```python
from build123d import *

# Parameters (mm, degrees)
SKETCH1_W           = 203.2
SKETCH1_H           = 152.4
BOSS_EXTRUDE1_DEPTH = 3.175


with BuildPart() as part:
    # Sketch1 → Boss-Extrude1 (new body)
    with BuildSketch(Plane(origin=(0, 0, 0), x_dir=(1, 0, 0), z_dir=(0, 1, 0))):
        with Locations((12.7, 0)):
            Rectangle(SKETCH1_W, SKETCH1_H)
        with BuildLine():
            Line((-48.396184338, 37.144491245), (-40.325508755, 43.316184338))
            ThreePointArc((-40.325508755, 43.316184338), (-33.204324417, 42.366693093), (-34.153815662, 35.245508755))
            Line((-34.153815662, 35.245508755), (-42.224491245, 29.073815662))
            ThreePointArc((-42.224491245, 29.073815662), (-49.345675583, 30.023306907), (-48.396184338, 37.144491245))
        make_face(mode=Mode.SUBTRACT)
        with BuildLine():
            Line((34.153815662, 35.245508755), (42.224491245, 29.073815662))
            ThreePointArc((42.224491245, 29.073815662), (49.345675583, 30.023306907), (48.396184338, 37.144491245))
            Line((48.396184338, 37.144491245), (40.325508755, 43.316184338))
            ThreePointArc((40.325508755, 43.316184338), (33.204324417, 42.366693093), (34.153815662, 35.245508755))
        make_face(mode=Mode.SUBTRACT)
        with BuildLine():
            Line((34.153815662, -35.245508755), (42.224491245, -29.073815662))
            ThreePointArc((42.224491245, -29.073815662), (49.345675583, -30.023306907), (48.396184338, -37.144491245))
            Line((48.396184338, -37.144491245), (40.325508755, -43.316184338))
            ThreePointArc((40.325508755, -43.316184338), (33.204324417, -42.366693093), (34.153815662, -35.245508755))
        make_face(mode=Mode.SUBTRACT)
        with BuildLine():
            Line((-48.396184338, -37.144491245), (-40.325508755, -43.316184338))
            ThreePointArc((-40.325508755, -43.316184338), (-33.204324417, -42.366693093), (-34.153815662, -35.245508755))
            Line((-34.153815662, -35.245508755), (-42.224491245, -29.073815662))
            ThreePointArc((-42.224491245, -29.073815662), (-49.345675583, -30.023306907), (-48.396184338, -37.144491245))
        make_face(mode=Mode.SUBTRACT)
    extrude(amount=BOSS_EXTRUDE1_DEPTH)


solid = part.part
```
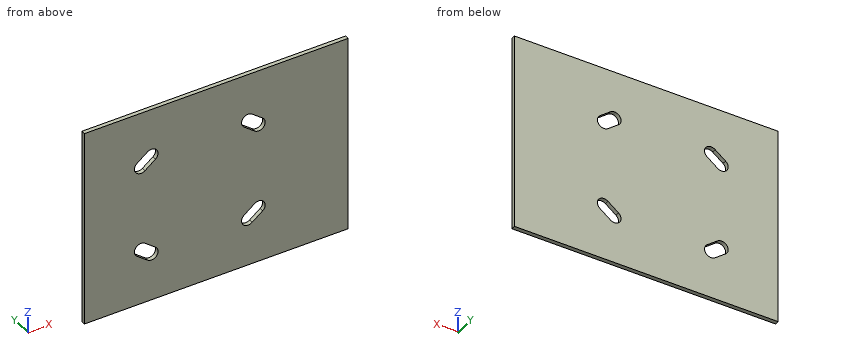
The listing builds one solid part. Answer for the finished solid, in the listing's coordinates (mm). Coordinates: 2 decimals unless noted, no trailing zeros. Write each loop counter-clockwise with the first axis right and the second up, starting at its lowest first coordinate (ties: lowest second). Pieces come first, ordered by that corner, then holes. Notation, with made-up numbers: (-9, 37.25) - (14, 37.25) arc R21 ccw to (14, 75.25) - close; hole circle Ø8 at (36.5, 57.25). An arc over 180 degrees is marked (long way). Return JSON: item names as keys, results as strings. Group by question number.
Q1. Find the intervals of material crossed by line 1 along Z through (x, y) = (36.5, 0.65); line 2 along Z through (x, y) = (-36, 1.95); line 3 along X through (y, z) = (2.4, 36), in increasing order. Write a range as [from, to].
Q2. The part is cut by section B-B on x = 36.5. Write down the section's boundary in (y, z) (3 decimals).
Q3. A flat-ended cylindrical pin translates along its axis: pin 1 Ø4 at (x, z) = (-11.5, -60) entering from -Y. Find the tip coordinate at first contact, or state that the pin passes through.
Q4. The part is cut by section A-A on y = 1.45. Write down the section's boundary in (x, z), and give its area (3 significant figures).
Evaluation:
{
 "1": {"line 1": "z = [-76.2, -44.31], [-33.45, 33.45], [44.31, 76.2]", "line 2": "z = [-76.2, -44.21], [-33.83, 33.83], [44.21, 76.2]", "line 3": "x = [-88.9, -49.49], [-33.36, 33.36], [49.49, 114.3]"},
 "2": {"outline": "(0, -76.2) - (3.175, -76.2) - (3.175, -44.307) - (0, -44.307) - close; (0, -33.451) - (3.175, -33.451) - (3.175, 33.451) - (0, 33.451) - close; (0, 44.307) - (3.175, 44.307) - (3.175, 76.2) - (0, 76.2) - close"},
 "3": {"pin 1": "stops at y = 0"},
 "4": {"outline": "(-88.9, -76.2) - (114.3, -76.2) - (114.3, 76.2) - (-88.9, 76.2) - close; hole (-48.4, -37.14) - (-40.33, -43.32) arc R5.08 ccw to (-34.15, -35.25) - (-42.22, -29.07) arc R5.08 ccw to start; hole (-48.4, 37.14) arc R5.08 ccw to (-42.22, 29.07) - (-34.15, 35.25) arc R5.08 ccw to (-40.33, 43.32) - close; hole (34.15, -35.25) arc R5.08 ccw to (40.33, -43.32) - (48.4, -37.14) arc R5.08 ccw to (42.22, -29.07) - close; hole (34.15, 35.25) - (42.22, 29.07) arc R5.08 ccw to (48.4, 37.14) - (40.33, 43.32) arc R5.08 ccw to start", "area": "30,200 mm2"}
}
